Can you work these out from the model? Positions are in its coordinate system, mm. A direction names the side the tool comes from. Coordinates: 2 decimals unless noted, no trailing zeros. Write each loop counter-clockwise with the first axis right and the second up, starting at its lowest first coordinate (ties: lowest second). Pieces come first, ordered by that corner, then holes.
```python
from build123d import *

# Parameters (mm, degrees)
BOSS_EXTRUDE1_DEPTH = 1.5


with BuildPart() as part:
    # Sketch1 → Revolve1 (revolve)
    with BuildSketch(Plane.XY):
        Polygon((0, 0), (1.9, 0), (1.9, 13), (2.825, 13), (2.825, 14.5), (0, 14.5), align=None)
    revolve(axis=Axis((0, 0, 0), (0, 1, 0)))

    # Sketch2 → Boss-Extrude1 (add, symmetric)
    with BuildSketch(Plane.XY):
        with BuildLine():
            Line((-2.325, 14.5), (-2.325, 21.45))
            ThreePointArc((-2.325, 21.45), (-1.314518395, 23.889518395), (1.125, 24.9))
            Line((1.125, 24.9), (1.225, 24.9))
            ThreePointArc((1.225, 24.9), (3.664518395, 23.889518395), (4.675, 21.45))
            Line((4.675, 21.45), (4.675, 15.5))
            Line((4.675, 15.5), (2.575, 15))
            Line((2.575, 15), (2.575, 14.5))
            Line((2.575, 14.5), (-2.325, 14.5))
        make_face()
    extrude(amount=BOSS_EXTRUDE1_DEPTH, both=True)

    # Sketch3 → DELETE CUT TO SEE REAL COMPONENT (revolve, cut)
    with BuildSketch(Plane.XY):
        Polygon((3.25, 15.5), (5.35, 17.8), (6.288787076, 17.8), (6.288787076, 14.5), (2.575, 14.5), (2.575, 14.913043478), align=None)
    revolve(axis=Axis((0, 0, 0), (0, 1, 0)), mode=Mode.SUBTRACT)


solid = part.part
```
1. We'd pull the mould along Y, two halves only. Please class faces 4 (the face through (2.842, 15.145, 0.025)), 5 (the face through (0, 0, 0)), 6 (the face through (-2.325, 18, 0)), 7 (the face through (3.638, 23.916, 0.021)): released by +Y, released by -Y, zero draft, split by the parting line, or undercut.
2. If I drill on L1, parallel to X at y = 17.25, z = -1 (3 decimals); L2, parallel to Y at x = 1, z = 0.9; L3, parallel to Z at x = 2.25, y = 21.5, over which ranges is the centre line in solid material (lowest first)?
3. Which directions (+Z, -Z, +X, -X, +Y, -Y) give clear straight access to the entire face, cutting with the end or side of a thin tool? Please do faces 1 (the face through (-1.9, 6.59, -0.08)), 2 (the face through (1, 20, 1.5)), 3 (the face through (1, 20, -1.5)).
4. If we section it at C-C, the plane z = 2.2: List the corners of the cut face in (x, y) for me.
5. If we section it at B-B, the plane x = 1.5: List the corners of the cut face in (y, z) for me, plus the area to 3 significant figures.
6. I'm going to push flat-ended pins straight in: P1, Ø3.5, axis at x = 0.5, y = 21, coming from the -Z side; P2, Ø3.5, axis at x = 0, y = 18.5, coming from the +Z side; P3, Ø1, axis at x = -1, y = 7.5, coming from the +Z side. Where does each tip first touch, or does it pass through?
7. If we section it at A-A, the plane y = 20: List the corners of the cut face in (x, z) for me (3 decimals), plus the area to 3 significant figures.
8. If we section it at D-D, the plane x = 0: List the corners of the cut face in (y, z) for me (3 decimals), plus the area to 3 significant figures.
Answers:
1. face 4: undercut
1. face 5: released by -Y
1. face 6: zero draft
1. face 7: released by +Y
2. L1: x = -2.325 to 4.675
2. L2: y = 0 to 24.9
2. L3: z = -1.5 to 1.5
3. face 1: -Y
3. face 2: +Z, +X, -X, +Y
3. face 3: -Z, +X, -X, +Y
4. outline: (-1.77, 13) - (1.77, 13) - (1.77, 14.5) - (-1.77, 14.5) - close
5. outline: (0, -1.17) - (13, -1.17) - (13, -2.39) - (14.5, -2.39) - (14.5, -1.5) - (24.89, -1.5) - (24.89, 1.5) - (14.5, 1.5) - (14.5, 2.39) - (13, 2.39) - (13, 1.17) - (0, 1.17) - close
5. area: 68.7 mm2
6. P1: stops at z = -1.5
6. P2: stops at z = 1.5
6. P3: stops at z = 1.83
7. outline: (-2.325, -1.5) - (4.675, -1.5) - (4.675, 1.5) - (-2.325, 1.5) - close
7. area: 21.0 mm2
8. outline: (0, -1.9) - (13, -1.9) - (13, -2.825) - (14.5, -2.825) - (14.5, -1.5) - (24.711, -1.5) - (24.711, 1.5) - (14.5, 1.5) - (14.5, 2.825) - (13, 2.825) - (13, 1.9) - (0, 1.9) - close
8. area: 88.5 mm2
